Answer from the drawing. Dimensions are ordinates in mm from the lowest x, y and z of the part. A direction names the side the tool comes from. Coordinates: 2 decimals unless noted, no trailing zeros. Order: outer loops, then holes, each group sorted by start corner. A loop starts at its lowest first (then second) coordinate and runs counter-clockwise, first axis right, second up. Notation, with made-up numbers: M 36,28.25 L 41,28.25 A7 ccw 41,32.25 Z; hole C -6.75,-5 d7. An arc over 180 degrees is marked long. Use a Markdown table: item, result.
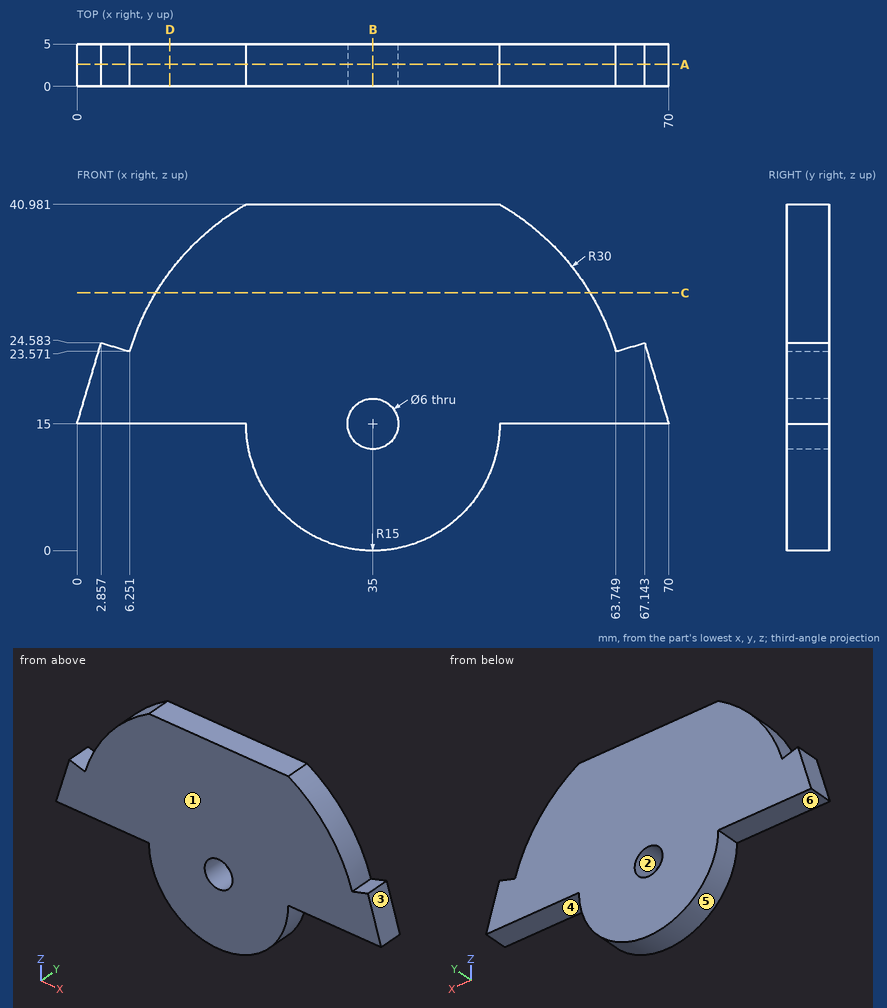
(1) A cutting plane is placed at A-A (y = 2.6). Determine the outline of the cut face in (x, z), then the cut area to 3 significant figures.
Conclusion:
| item | result |
|---|---|
| outline | M 0,15 L 20,15 A15 ccw 50,15 L 70,15 L 67.14,24.58 L 63.75,23.57 A30 ccw 50,40.98 L 20,40.98 A30 ccw 6.25,23.57 L 2.86,24.58 Z; hole C 35,15 d6 |
| area | 1,730 mm2 |
(2) A cutting plane is placed at D-D (x = 11). Determine the outline of the cut face in (y, z), then the cut area to 3 significant figures.
Conclusion:
| item | result |
|---|---|
| outline | M 0,15 L 5,15 L 5,33 L 0,33 Z |
| area | 90.0 mm2 |
(3) A cutting plane is placed at B-B (x = 35). Determine the outline of the cut face in (y, z), then the cut area to 3 significant figures.
Conclusion:
| item | result |
|---|---|
| outline | M 0,0 L 5,0 L 5,12 L 0,12 Z; M 0,18 L 5,18 L 5,40.98 L 0,40.98 Z |
| area | 175 mm2 |
(4) Which of the six approach directions +Z, -Z, +X, -X, +Y, -Y give full straight-line access (tool end or side, diameter ignored) to the marked faces 4, 5 and 6?
Conclusion:
| item | result |
|---|---|
| face 4 | -Z, +X, +Y, -Y |
| face 5 | -Z, +Y, -Y |
| face 6 | -Z, -X, +Y, -Y |
(5) Straight lines are drawn through the part: L1, parallel to Z at x = 35, y = 1.55; L2, parallel to Z at x = 8.5, y = 2.25 (1 decimal); L3, parallel to X at y = 4.7, z = 30. For each, find the intervals that lie inside material, in ascending order.
Conclusion:
| item | result |
|---|---|
| L1 | 0 to 12, 18 to 40.98 |
| L2 | 15 to 29.1 |
| L3 | 9.02 to 60.98 |
(6) Given P1, Ø3, axis at y = 1, z = 33.5, coming from the -X side; P2, Ø1.5, axis at x = 63, y = 1.5, coming from the -Z side; P3, Ø1.5, axis at y = 4, z = 24.5, coming from the +X side, each flat-ended and moving along its own axis, determine where each tip first touches the part or whether it passes through.
Conclusion:
| item | result |
|---|---|
| P1 | x = 10.28 |
| P2 | z = 15 |
| P3 | x = 67.39 |
(7) Determine the mould class of the marked faces 1, 2 and 3 for opening direction X: pulls with the +X half, pulls with the -X half, needs draft (parallel to the pull), parting line crosses it, or undercut.
Conclusion:
| item | result |
|---|---|
| face 1 | needs draft |
| face 2 | undercut |
| face 3 | pulls with the +X half |
(8) A cutting plane is placed at C-C (z = 30.5). Determine the outline of the cut face in (x, y) (1 decimal), then the cut area to 3 significant figures.
Conclusion:
| item | result |
|---|---|
| outline | M 9.3,0 L 60.7,0 L 60.7,5 L 9.3,5 Z |
| area | 257 mm2 |
